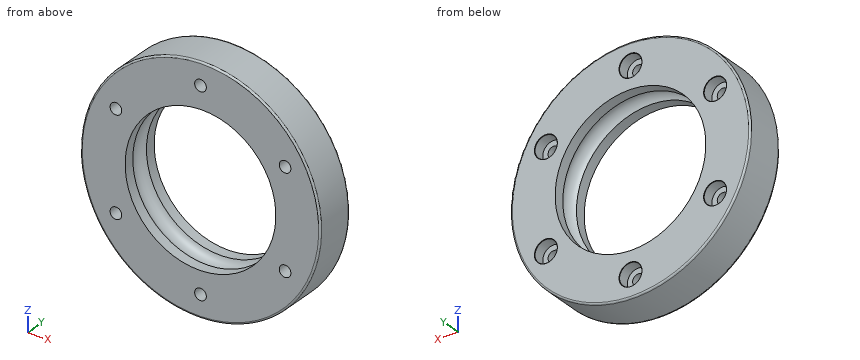
```python
from build123d import *

# Parameters (mm, degrees)
FILLET_1_R          = 0.5
SKETCH_2_R          = 1.7
CUT_EXTRUDE_1_DEPTH = 20
SKETCH_3_R          = 3.25
CUT_EXTRUDE_2_DEPTH = 3.3
CHAMFER_1_SIZE      = 0.1


with BuildPart() as part:
    # 草图1 → 旋转1 (revolve)
    with BuildSketch(Plane.XY, mode=Mode.PRIVATE) as revolve_1_sk:
        with BuildLine():
            Line((-22, 6), (-22, 2.828427125))
            ThreePointArc((-22, 2.828427125), (-24, 0), (-22, -2.828427125))
            Line((-22, -2.828427125), (-22, -6))
            Line((-22, -6), (-35, -6))
            Line((-35, -6), (-35, 6))
            Line((-35, 6), (-22, 6))
        make_face()
    revolve(revolve_1_sk.sketch.rotate(Axis((0, 15.876951414, 0), (0, -1, 0)), 270), axis=Axis((0, 15.876951414, 0), (0, -1, 0)))

    # 圆角1
    fillet_1_edges = [part.edges().sort_by_distance(p)[0] for p in [
        (0, -6, -35),
        (0, 6, -35),
    ]]
    fillet(fillet_1_edges, radius=FILLET_1_R)

    # 草图2 → 切除-拉伸1 (cut)
    with BuildSketch(Plane(origin=(0, 6, 0), x_dir=(1, 0, 0), z_dir=(0, 1, 0))):
        with Locations(Location((0, 28.5, 0), (0, 0, 270))):
            Circle(SKETCH_2_R)
        with Locations(Location((24.681724008, 14.25, 0), (0, 0, 270))):
            Circle(SKETCH_2_R)
        with Locations(Location((24.681724008, -14.25, 0), (0, 0, 270))):
            Circle(SKETCH_2_R)
        with Locations(Location((0, -28.5, 0), (0, 0, 270))):
            Circle(SKETCH_2_R)
        with Locations(Location((-24.681724008, -14.25, 0), (0, 0, 270))):
            Circle(SKETCH_2_R)
        with Locations(Location((-24.681724008, 14.25, 0), (0, 0, 270))):
            Circle(SKETCH_2_R)
    extrude(amount=-CUT_EXTRUDE_1_DEPTH, mode=Mode.SUBTRACT)

    # 草图3 → 切除-拉伸2 (cut)
    with BuildSketch(Plane(origin=(0, 6, 0), x_dir=(1, 0, 0), z_dir=(0, 1, 0))):
        with Locations(Location((0, 28.5, 0), (0, 0, 270))):
            Circle(SKETCH_3_R)
        with Locations(Location((24.681724008, 14.25, 0), (0, 0, 270))):
            Circle(SKETCH_3_R)
        with Locations(Location((24.681724008, -14.25, 0), (0, 0, 270))):
            Circle(SKETCH_3_R)
        with Locations(Location((0, -28.5, 0), (0, 0, 270))):
            Circle(SKETCH_3_R)
        with Locations(Location((-24.681724008, -14.25, 0), (0, 0, 270))):
            Circle(SKETCH_3_R)
        with Locations(Location((-24.681724008, 14.25, 0), (0, 0, 270))):
            Circle(SKETCH_3_R)
    extrude(amount=-CUT_EXTRUDE_2_DEPTH, mode=Mode.SUBTRACT)

    # 倒角1
    chamfer_1_edges = [part.edges().sort_by_distance(p)[0] for p in [
        (0, 6, -31.75),
        (24.681724008, 6, -17.5),
        (24.681724008, 6, 11),
        (0, 6, 25.25),
        (-24.681724008, 6, 11),
        (-24.681724008, 6, -17.5),
    ]]
    chamfer(chamfer_1_edges, length=CHAMFER_1_SIZE)


solid = part.part
```
Input: part model. Units: mm. Frame: model coordinates. Coordinates: 2 decimals unless noted, no trailing zeros. Loops run counter-clockwise (first coordinate to the right, second up) from the corner with the lowest first, then second, coordinate; pieces in that order, holes last.
Q1. Line query: line 1 along X through (y, z) = (-3, -14.25); line 2 along X through (y, z) = (3.5, -12); line 3 along Z through (x, y) = (26, 0.5). Output: solid intervals per line, ascending.
Results are:
line 1: x = -31.97 to -26.38, -22.98 to -16.76, 16.76 to 22.98, 26.38 to 31.97
line 2: x = -32.88 to -27.03, -22.34 to -18.44, 18.44 to 22.34, 27.03 to 32.88
line 3: z = -23.43 to -15.32, -13.18 to 13.18, 15.32 to 23.43
Q2. Section B-B, the plane x = 0. Give the number of separate pieces and of enclosed holes in the cut face, and give its area (3 significant figures).
Results are:
separate pieces: 4
enclosed holes: 0
area: 193 mm2
Q3. Section C-C, the plane y = 4. Return the cut outline in (x, z), and give its area (3 significant figures).
Results are:
outline: circle Ø70 at (0, 0); hole circle Ø6.5 at (-24.68, -14.25); hole circle Ø6.5 at (-24.68, 14.25); hole circle Ø44 at (0, 0); hole circle Ø6.5 at (0, -28.5); hole circle Ø6.5 at (0, 28.5); hole circle Ø6.5 at (24.68, -14.25); hole circle Ø6.5 at (24.68, 14.25)
area: 2,130 mm2
Q4. Section A-A, the plane z = 0. Return the cut outline in (x, y), and give its area (3 significant figures).
Results are:
outline: (-35, -5.5) arc R0.5 ccw to (-34.5, -6) - (-22, -6) - (-22, -2.83) arc R3 cw to (-22, 2.83) - (-22, 6) - (-34.5, 6) arc R0.5 ccw to (-35, 5.5) - close; (22, -6) - (34.5, -6) arc R0.5 ccw to (35, -5.5) - (35, 5.5) arc R0.5 ccw to (34.5, 6) - (22, 6) - (22, 2.83) arc R3 cw to (22, -2.83) - close
area: 295 mm2
Q5. Contact query for flat-ended pins moving along their axis: pin 1 (3 mm diameter, centred on x = -24.68, z = -14.25, fed in from +Y); pin 2 (2 mm diameter, centred on x = 1, z = 29.5, fed in from +Y); pin 3 (2 mm diameter, centred on y = -4.5, z = 17, fed in from -X); pin 4 (1 mm diameter, centred on x = 23, y = -0.5, fed in from +Z). Output: stop coordinate, or through.
Results are:
pin 1: passes through
pin 2: stops at y = 2.7
pin 3: stops at x = -31.13
pin 4: stops at z = 26.81
